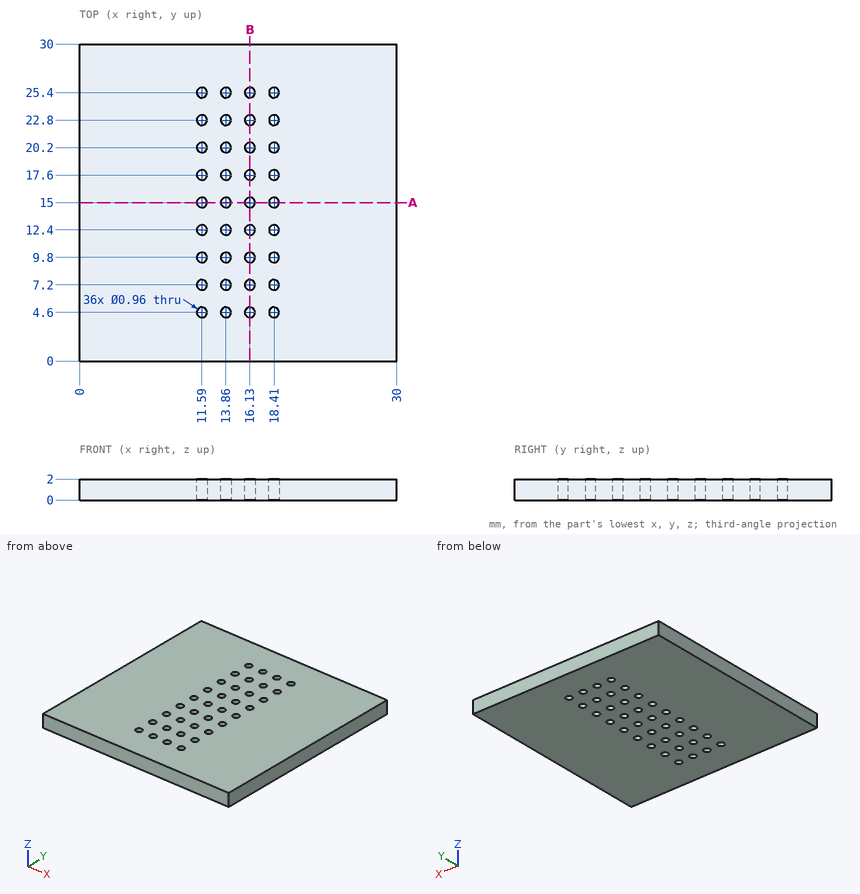
Source: three-view drawing plus pictorial views. Frame: mm from the lowest corner of the part. Give positions to 0.01 mm unless a question says otherwise; leave off trailing zeros. Order: outer loops, then holes, each group sorted by start corner. A loop starts at its lowest first (then second) coordinate and runs counter-clockwise, first axis right, second up. Notation, with made-up numbers: M -29,71.25 L -5,71.25 A21 ccw -5,110.25 Z; hole C -35.75,-31 d2. An arc over 180 degrees is marked long. One line per question, with ' | ' between items. Start each with the question number.
1. Section query B-B (x = 16.13). Count the separate pieces of the cut face and the enclosed holes in it, and give its area (3 significant figures).
2. Material intervals for probe 1 along X at (y, z) = (4.5, 0.9); probe 2 along X at (y, z) = (9.5, 1.65), sorted ascending. Write a range as [from, to].
3. Section query A-A (y = 15). Return the cut outline in (x, z), and give its area (3 significant figures).
Here are the results:
1) separate pieces: 10 | enclosed holes: 0 | area: 42.7 mm²
2) probe 1: [0, 11.12], [12.06, 13.39], [14.33, 15.66], [16.6, 17.94], [18.88, 30] | probe 2: [0, 11.22], [11.96, 13.49], [14.23, 15.76], [16.5, 18.04], [18.78, 30]
3) outline: M 0,0 L 11.11,0 L 11.11,2 L 0,2 Z; M 12.07,0 L 13.38,0 L 13.38,2 L 12.07,2 Z; M 14.34,0 L 15.65,0 L 15.65,2 L 14.34,2 Z; M 16.61,0 L 17.93,0 L 17.93,2 L 16.61,2 Z; M 18.89,0 L 30,0 L 30,2 L 18.89,2 Z | area: 52.3 mm²
